Geometry check sheet. Reference: the model listing, model coordinates, mm. Face numbers are marked on the shaded views. A direction names the side the tool comes from. Coordinates: 2 decimals unless noted, no trailing zeros. Order: outer loops, then holes, each group sorted by start corner. A loop starts at its lowest first (then second) coordinate and runs counter-clockwise, first axis right, second up. Notation, with made-up numbers: (17.25, 23) - (22.25, 23) arc R23 ccw to (22.25, 37) - close; hole circle Ø8 at (70, -25). An arc over 180 degrees is marked (long way). Return JSON: item names as keys, results as strings. Group by question number.
Item 1: Section check B-B on x = 0. Enter the section's corners in (y, z).
Item 2: Scan lines: probe 1 along Z at (x, y) = (0, 78.5); probe 2 along Y at (x, z) = (10.5, -6); probe 3 along Y at (x, z) = (10.5, 21.5). Record each from-to range of solid material in increasing order.
Item 3: Section check C-C on y = 52. Enter the section's corners in (x, z).
Item 4: Section check A-A on z = 0. Enter the section's corners in (x, y), then the cut area to 3 significant figures.
Item 5: Gauge pin test, flat ends, axial feed: pin 1 (1 mm diameter, centred on x = 16, z = 20, fed in from -Y); pin 2 (8 mm diameter, centred on x = -6.5, y = 39, fed in from -Z); pin 3 (5 mm diameter, centred on x = -12.5, y = 79, fed in from -Z). Record the tip position at first contact, or that the pin passes through.
Item 6: Section check D-D on x = 8.5. Enter the section's corners in (y, z), then the cut area to 3 significant figures.
Item 7: Tool access check on the marked faces 1, 2 and 3. Record the directions out of +Z, -Z, +X, -X, +Y, -Y that give a thin tool (end or side, any length) a straight path to the whole face; none if there is none.
Autodesk Inventor part; units mm, degrees
ref_plane "YZ Plane" through (0, 0, 0) normal (1, 0, 0) x (0, 1, 0)
ref_plane "XZ Plane" through (0, 0, 0) normal (0, 1, 0) x (-1, 0, 0)
ref_plane "XY Plane" through (0, 0, 0) normal (0, 0, 1) x (1, 0, 0)
sketch "Sketch1" plane through (0, 0, 0) normal (0, 1, 0) x (-1, 0, 0)
  circle A0 centre (0, 0) radius 20.1549
  dimension "d0" = 40.3098
extrude "Extrusion1" add sketch "Sketch1" along normal blind 58.2676
sketch "Sketch2" plane through (0, 58.2676, 0) normal (0, 1, 0) x (1, 0, 0)
  circle A0 centre (0, 0) radius 29.21
  dimension "d3" = 58.42
extrude "Extrusion2" add sketch "Sketch2" along normal blind 34.7726
sketch "Sketch3" plane through (0, 93.0402, 0) normal (0, 1, 0) x (1, 0, 0)
  circle A0 centre (0, 0) radius 14.3002
  dimension "d6" = 28.6004
extrude "Extrusion3" add sketch "Sketch3" along normal blind 1.8288
sketch "Sketch4" plane through (0, 93.0402, 0) normal (0, 1, 0) x (1, 0, 0)
  circle A0 centre (0, 20.7518) radius 1.905
  circle A1 centre (0, 0) radius 14.3002
  line L0 (-34.2978, 0) -> (34.9424, 0) construction
  circle A2 centre (0, -20.7518) radius 1.905
  dimension "d9" = 3.81
  dimension "d10" = 4.5466
extrude "Extrusion4" cut sketch "Sketch4" against normal blind 33.02 contours A0 | A2
sketch "Sketch5" plane through (0, 94.869, 0) normal (0, 1, 0) x (1, 0, 0)
  circle A0 centre (8.6926, 0) radius 3.1877
  point P0 (0, 0)
  dimension "d13" = 6.3754
  dimension "d14" = 8.6926
extrude "Extrusion5" add sketch "Sketch5" along normal blind 17.78
sketch "Sketch6" plane through (8.6926, 112.649, 0) normal (0, 1, 0) x (1, 0, 0)
  circle A0 centre (0, 0) radius 3.1877
  line L0 (-1.8509, -2.5953) -> (-1.8509, 2.5953)
  arc A1 (-1.8509, 2.5953) -> (-1.8509, -2.5953) centre (0, 0) ccw
  point P0 (-8.6926, 0)
extrude "Extrusion6" cut sketch "Sketch6" against normal blind 17.78 contours L0 A0 picked at (-2.2965, 0)
properties part number "Autofeeder motor"
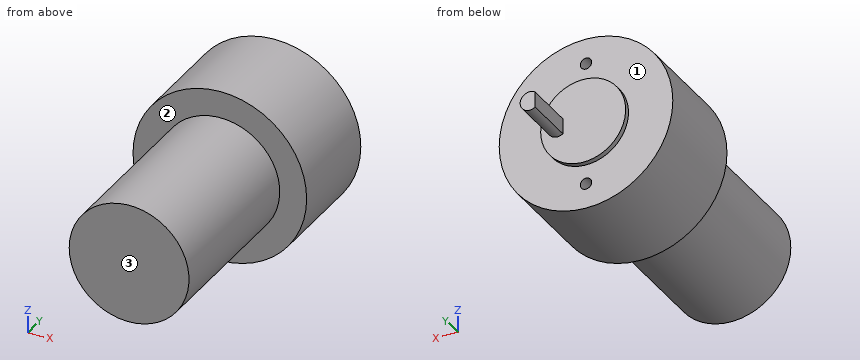
Computed:
{
 "1": {"outline": "(0, -20.15) - (58.27, -20.15) - (58.27, -29.21) - (93.04, -29.21) - (93.04, -22.66) - (60.02, -22.66) - (60.02, -18.85) - (93.04, -18.85) - (93.04, -14.3) - (94.87, -14.3) - (94.87, 14.3) - (93.04, 14.3) - (93.04, 18.85) - (60.02, 18.85) - (60.02, 22.66) - (93.04, 22.66) - (93.04, 29.21) - (58.27, 29.21) - (58.27, 20.15) - (0, 20.15) - close"},
 "2": {"probe 1": "z = -29.21 to -22.66, -18.85 to 18.85, 22.66 to 29.21", "probe 2": "y = 0 to 94.87", "probe 3": "y = 58.27 to 93.04"},
 "3": {"outline": "circle Ø40.31 at (0, 0)"},
 "4": {"outline": "(-29.21, 58.27) - (-20.15, 58.27) - (-20.15, 0) - (20.15, 0) - (20.15, 58.27) - (29.21, 58.27) - (29.21, 93.04) - (14.3, 93.04) - (14.3, 94.87) - (11.88, 94.87) - (11.88, 112.65) - (6.84, 112.65) - (6.84, 94.87) - (-14.3, 94.87) - (-14.3, 93.04) - (-29.21, 93.04) - close", "area": "4,520 mm²"},
 "5": {"pin 1": "stops at y = 58.27", "pin 2": "stops at z = -20", "pin 3": "stops at z = -27.44"},
 "6": {"outline": "(0, -18.27) - (58.27, -18.27) - (58.27, -27.95) - (93.04, -27.95) - (93.04, -11.5) - (94.87, -11.5) - (94.87, -3.18) - (112.65, -3.18) - (112.65, 3.18) - (94.87, 3.18) - (94.87, 11.5) - (93.04, 11.5) - (93.04, 27.95) - (58.27, 27.95) - (58.27, 18.27) - (0, 18.27) - close", "area": "4,230 mm²"},
 "7": {"face 1": "+Y", "face 2": "-Y", "face 3": "+Z, -Z, +X, -X, -Y"}
}
